Input: part model. Units: mm. Frame: model coordinates. Face numbers are marked on the shaded views. A direction names the side the tool comes from. Give positions to 0.01 mm unless a question says otherwise; leave off trailing zeros. Write each loop counter-clockwise with the first axis right and the second up, starting at its lowest first coordinate (ties: lowest second). Pieces come first, ordered by that corner, then holes. Notation, with made-up numbers: (51, -39.75) - (55, -39.75) arc R26 ccw to (55, -7.75) - close; hole circle Ø10 at (69.25, 32.5). An arc over 180 degrees is marked (long way). Use a Markdown table: item, result. Add a question column.
1. Material intervals for probe 1 along Z at (x, y) = (1.5, 8); probe 2 along Z at (x, y) = (20, 0.9); probe 3 along Y at (x, z) = (10, -28.25), sorted ascending.
2. Set-up query: the marked faces 1 and 2. Return all of +Z, -Z, +X, -X, +Y, -Y with unobstructed straight access to the full face (end or side cutting, diameter ignored); none if empty.
3. Section query A-A, the plane z = -15. Return loops of the section in (x, y), plus the area to 3 significant figures.
4. Section query B-B, the plane y = 8. Return loops of the section in (x, z).
5. Section query D-D, the plane z = -23.25. Return loops of the section in (x, y).
6. Section query C-C, the plane x = 22.5. Return loops of the section in (y, z), plus the area to 3 significant figures.
7. Pin query (flat end, axial travel): pin 1 (8 mm diameter, centred on y = 5, z = -19, fed in from +X). Return the tip coordinate at first contact, or that it passes through.
```python
from build123d import *

# Parameters (mm, degrees)
BOSS_EXTRUDE1_DEPTH     = 30
EXTRUDE_THIN1_DEPTH     = 2
SKETCH3_R               = 9
CUT_EXTRUDE1_DEPTH      = 48.634021455
FILLET2_R               = 4
CUT_EXTRUDE2_DEPTH      = 49.176757882
CUT_EXTRUDE2_DEPTH_BACK = 49.176757882
SKETCH4_R               = 2
FILLET3_R               = 2


with BuildPart() as part:
    # Sketch1 → Boss-Extrude1 (new body)
    with BuildSketch(Plane.XY):
        Polygon((0, 0), (20, 0), (20, 2), (2, 2), (2, 14), (0, 14), align=None)
    extrude(amount=-BOSS_EXTRUDE1_DEPTH)

    # Sketch2 → Extrude-Thin1 (add)
    with BuildSketch(Plane(origin=(0, 0, 0), x_dir=(1, 0, 0), z_dir=(0, 1, 0))):
        with BuildLine():
            ThreePointArc((20, 30), (35, 15), (20, 0))
            Line((20, 0), (20, 10))
            ThreePointArc((20, 10), (25, 15), (20, 20))
            Line((20, 20), (20, 30))
        make_face()
    extrude(amount=EXTRUDE_THIN1_DEPTH)

    # Sketch3 → Cut-Extrude1 (cut, through all)
    with BuildSketch(Plane(origin=(0, 2, 0), x_dir=(1, 0, 0), z_dir=(0, 1, 0))):
        with Locations(Location((20, 15, 0), (0, 0, 180))):
            Circle(SKETCH3_R)
    extrude(amount=-CUT_EXTRUDE1_DEPTH, mode=Mode.SUBTRACT)

    # Fillet2
    fillet2_edges = [part.edges().sort_by_distance(p)[0] for p in [
        (0, 0, -15),
    ]]
    fillet(fillet2_edges, radius=FILLET2_R)

    # Sketch4 → Cut-Extrude2 (cut, two sides: drawn at the far end of the back side and taken through both)
    with BuildSketch(Plane(origin=(0, 0, 0), x_dir=(0, 0, -1), z_dir=(1, 0, 0)).offset(-CUT_EXTRUDE2_DEPTH_BACK)):
        with Locations((15, 8)):
            Circle(SKETCH4_R)
    extrude(amount=CUT_EXTRUDE2_DEPTH + CUT_EXTRUDE2_DEPTH_BACK, mode=Mode.SUBTRACT)

    # Fillet3
    fillet3_edges = [part.edges().sort_by_distance(p)[0] for p in [
        (1, 14, -30),
        (1, 14, 0),
    ]]
    fillet(fillet3_edges, radius=FILLET3_R)


solid = part.part
```
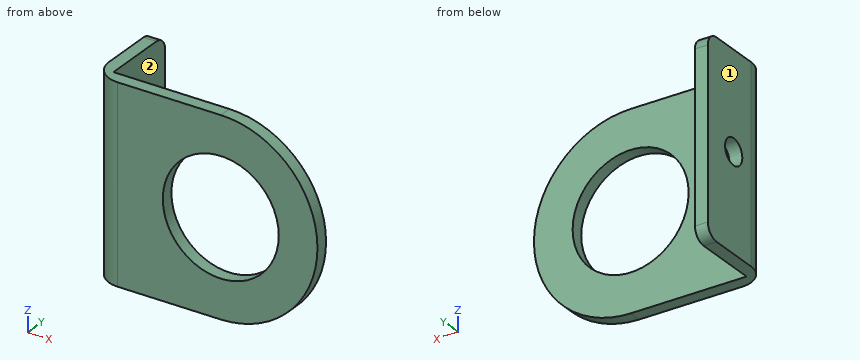
Result sheet:
| question | item | result |
|---|---|---|
| 1 | probe 1 | z = -30 to -17, -13 to 0 |
| 1 | probe 2 | z = -30 to -24, -6 to 0 |
| 1 | probe 3 | y = 0 to 2 |
| 2 | face 1 | +Z, -Z, -X, +Y, -Y |
| 2 | face 2 | +Z, -Z, +X, +Y |
| 3 | outline | (0, 4) arc R4 ccw to (4, 0) - (11, 0) - (11, 2) - (2, 2) - (2, 6) - (0, 6) - close; (0, 10) - (2, 10) - (2, 14) - (0, 14) - close; (29, 0) - (35, 0) - (35, 2) - (29, 2) - close |
| 3 | area | 46.6 mm² |
| 4 | outline | (0, -30) - (2, -30) - (2, -17) - (0, -17) - close; (0, -13) - (2, -13) - (2, 0) - (0, 0) - close |
| 5 | outline | (0, 4) arc R4 ccw to (4, 0) - (16.4, 0) - (16.4, 2) - (2, 2) - (2, 14) - (0, 14) - close; (23.6, 0) - (32.53, 0) - (32.53, 2) - (23.6, 2) - close |
| 6 | outline | (0, -29.79) - (2, -29.79) - (2, -23.65) - (0, -23.65) - close; (0, -6.35) - (2, -6.35) - (2, -0.21) - (0, -0.21) - close |
| 6 | area | 24.6 mm² |
| 7 | pin 1 | stops at x = 34.94 |
